Geometry check sheet. Reference: the model listing, model coordinates, mm. A direction names the side the tool comes from. Coordinates: 2 decimals unless noted, no trailing zeros. Order: outer loops, then holes, each group sorted by start corner. A loop starts at its lowest first (then second) coordinate and runs counter-clockwise, first axis right, second up. Notation, with made-up numbers: M -19.75,-6 L 20.25,-6 A19 ccw 20.25,30 Z; hole C 20,59 d6. An arc over 180 degrees is marked long. One line per item, written item: value. Start each with the question number.
1) Draft check along Z on faces 1 (the cylindrical face through (-7.7, 1.4, -10.1)), 2 (the cylindrical face through (0.767, 93.229, -2.435)), 3 (the flat face through (0, -101.6, 3)). Enter one of: pulls with the +Z half, pulls with the -Z half, needs draft (parallel to the pull), parting line crosses it, or undercut.
2) Access from +Z, -Z, +X, -X, +Y, -Y to the whole of each face (thin tool, end or side, straight path). Record for faces 4 (the cylindrical face through (0.767, -93.229, 2.435)), 5 (the flat face through (0, 101.6, 3)).
3) Sectioned sample at C-C, the plane x = -10.25. Enter the section's corners in (y, z), then the cut area to 3 significant figures.
4) Sectioned sample at A-A, the plane y = -47. Enter the section's corners in (x, z), then the cut area to 3 significant figures.
5) Go/stop test with flat-tipped pins: P1, Ø1.5, axis at x = 5.5, y = -80.5, coming from the -Z side; P2, Ø1, axis at y = -70.5, z = 6.5, coming from the +X side; P3, Ø4, axis at x = 0, z = 0, coming from the +Y side. Record where each tip stops, or that it passes through.
6) Thickness scan on L1, parallel to X at y = -90.5, z = 0; L2, parallel to Z at x = -9.5, y = 55. Record the ranges inside material, lowest first. Write a range as from..to.
7) Sectioned sample at B-B, the plane z = -11. Enter the section's corners in (x, y).
```python
from build123d import *

# Parameters (mm, degrees)
SKETCH1_R                             = 12.7
BOSS_EXTRUDE1_DEPTH                   = 101.6
F_1_4_20_TAPPED_HOLE1_D               = 5.1054
F_1_4_20_TAPPED_HOLE1_DEPTH           = 16.51
F_1_4_20_TAPPED_HOLE1_TIP             = 1.533816902
F_1_4_20_TAPPED_HOLE1_ON_FACE_2_D     = 5.1054
F_1_4_20_TAPPED_HOLE1_ON_FACE_2_DEPTH = 16.51
F_1_4_20_TAPPED_HOLE1_ON_FACE_2_TIP   = 1.533816902


with BuildPart() as part:
    # Sketch1 → Boss-Extrude1 (new, symmetric)
    with BuildSketch(Plane(origin=(0, 0, 0), x_dir=(1, 0, 0), z_dir=(0, 1, 0))):
        with Locations(Location((0, 0, 0), (0, 0, 270))):
            Circle(SKETCH1_R)
    extrude(amount=BOSS_EXTRUDE1_DEPTH, both=True)

    # 1/4-20 Tapped Hole1
    with Locations(Plane.ZX.offset(101.6)):
        with Locations((0, 0)):
            Hole(F_1_4_20_TAPPED_HOLE1_D / 2, depth=F_1_4_20_TAPPED_HOLE1_DEPTH)
            with Locations((0, 0, -(F_1_4_20_TAPPED_HOLE1_DEPTH + F_1_4_20_TAPPED_HOLE1_TIP / 2))):  # 118° drill point
                Cone(0, F_1_4_20_TAPPED_HOLE1_D / 2, F_1_4_20_TAPPED_HOLE1_TIP, mode=Mode.SUBTRACT)

    # 1/4-20 Tapped Hole1 on face 2
    with Locations(Plane(origin=(0, -101.6, 0), x_dir=(0, 0, -1), z_dir=(0, -1, 0))):
        with Locations((0, 0)):
            Hole(F_1_4_20_TAPPED_HOLE1_ON_FACE_2_D / 2, depth=F_1_4_20_TAPPED_HOLE1_ON_FACE_2_DEPTH)
            with Locations((0, 0, -(F_1_4_20_TAPPED_HOLE1_ON_FACE_2_DEPTH + F_1_4_20_TAPPED_HOLE1_ON_FACE_2_TIP / 2))):  # 118° drill point
                Cone(0, F_1_4_20_TAPPED_HOLE1_ON_FACE_2_D / 2, F_1_4_20_TAPPED_HOLE1_ON_FACE_2_TIP, mode=Mode.SUBTRACT)


solid = part.part
```
Final values:
1. face 1: parting line crosses it
1. face 2: undercut
1. face 3: needs draft
2. face 4: -Y
2. face 5: +Z, -Z, +X, -X, +Y
3. outline: M -101.6,-7.5 L 101.6,-7.5 L 101.6,7.5 L -101.6,7.5 Z
3. area: 3,050 mm^2
4. outline: C 0,0 d25.4
4. area: 507 mm^2
5. P1: stops at z = -11.78
5. P2: stops at x = 11.19
5. P3: stops at y = 84.76
6. L1: x = -12.7..-2.55, 2.55..12.7
6. L2: z = -8.43..8.43
7. outline: M -6.35,-101.6 L 6.35,-101.6 L 6.35,101.6 L -6.35,101.6 Z
